from build123d import *

# Parameters (mm, degrees)
F1_DEPTH = 100
F3_DEPTH = 100.001
F5_D     = 9


with BuildPart() as f1:
    # F0 (on Top) → F1 (new body)
    with BuildSketch(Plane.XY):
        with BuildLine():
            ThreePointArc((22, 17), (20.535534, 20.535534), (17, 22))
            Line((17, 22), (-17, 22))
            ThreePointArc((-17, 22), (-20.535534, 20.535534), (-22, 17))
            Line((-22, 17), (-22, -17))
            ThreePointArc((-22, -17), (-20.535534, -20.535534), (-17, -22))
            Line((-17, -22), (17, -22))
            ThreePointArc((17, -22), (20.535534, -20.535534), (22, -17))
            Line((22, -17), (22, 17))
        make_face()
    extrude(amount=F1_DEPTH)

    # F2 (on face) → F3 (cut, through all)
    with BuildSketch(Plane.XY.offset(100)):
        with BuildLine():
            ThreePointArc((-19, -17), (-18.414214, -18.414214), (-17, -19))
            Line((-17, -19), (17, -19))
            ThreePointArc((17, -19), (18.414214, -18.414214), (19, -17))
            Line((19, -17), (19, 17))
            ThreePointArc((19, 17), (18.414214, 18.414214), (17, 19))
            Line((17, 19), (-17, 19))
            ThreePointArc((-17, 19), (-18.414214, 18.414214), (-19, 17))
            Line((-19, 17), (-19, -17))
        make_face()
    extrude(amount=-F3_DEPTH, mode=Mode.SUBTRACT)

    # F5 (through all)
    with Locations(Plane.YZ.offset(22)):
        with Locations((0, 50)):
            Hole(F5_D / 2)


solid = f1.part
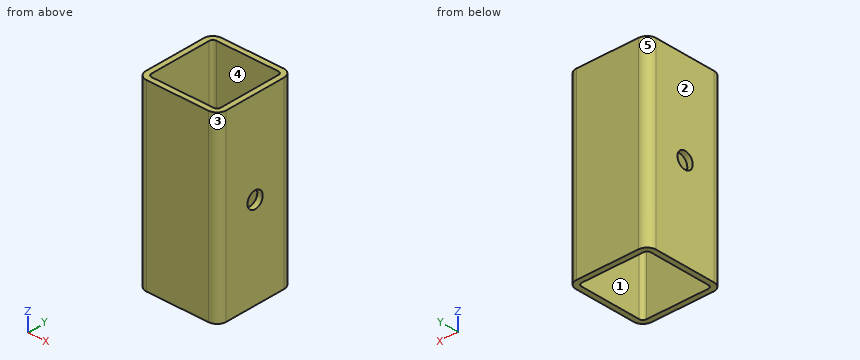
Here's how the part is built. I have some questions about the finished solid (model axes, mm). Face numbers are marked on the shaded views. A direction names the side the tool comes from. Round coordinates to 2 decimals unless told otherwise and drop trailing zeros. Write each loop counter-clockwise with the first axis right and the second up, starting at its lowest first coordinate (ties: lowest second). Pieces come first, ordered by that corner, then holes.
1. Suppose I cut it at D-D (z = 74). List the corners of the cut face in (x, y) for me.
2. For the marked faces 4 and 5, which set-ups out of +Z, -Z, +X, -X, +Y, -Y let a thin tool reach every point of the face, with its end or its side?
3. If we mould it in two halves opening along X, with no side actions, what happens to the marked faces 1, 2 and 3? For each: released by +X, released by -X, zero draft, split by the parting line, or undercut.
4. I need wall thicknesses on L1, parallel to Y at x = 15.5, z = 40; L2, parallel to Z at x = 20.6, y = 0. Which ranges of each line are inside material? Lowest first, please.
5. Suppose I cut it at B-B (y = 8.5). List the corners of the cut face in (x, z) for me.
6. Suppose I cut it at A-A (z = 50). List the corners of the cut face in (x, y) for me, and give its area (3 significant figures).
7. Will this pin go through, and if not, where does the flat tip stop? pin 1 Ø8 at (y, z) = (0, 50) entering from -X.
Answer sheet:
1. outline: (-22, -17) arc R5 ccw to (-17, -22) - (17, -22) arc R5 ccw to (22, -17) - (22, 17) arc R5 ccw to (17, 22) - (-17, 22) arc R5 ccw to (-22, 17) - close; hole (-19, -17) arc R2 ccw to (-17, -19) - (17, -19) arc R2 ccw to (19, -17) - (19, 17) arc R2 ccw to (17, 19) - (-17, 19) arc R2 ccw to (-19, 17) - close
2. face 4: +Z, -Z
2. face 5: +Z, -Z, -X, +Y
3. face 1: undercut
3. face 2: released by -X
3. face 3: released by +X
4. L1: y = -22 to -19, 19 to 22
4. L2: z = 0 to 45.5, 54.5 to 100
5. outline: (-22, 0) - (-19, 0) - (-19, 100) - (-22, 100) - close; (19, 0) - (22, 0) - (22, 100) - (19, 100) - close
6. outline: (-22, -17) arc R5 ccw to (-17, -22) - (17, -22) arc R5 ccw to (22, -17) - (22, -4.5) - (19, -4.5) - (19, -17) arc R2 cw to (17, -19) - (-17, -19) arc R2 cw to (-19, -17) - (-19, -4.5) - (-22, -4.5) - close; (-22, 4.5) - (-19, 4.5) - (-19, 17) arc R2 cw to (-17, 19) - (17, 19) arc R2 cw to (19, 17) - (19, 4.5) - (22, 4.5) - (22, 17) arc R5 ccw to (17, 22) - (-17, 22) arc R5 ccw to (-22, 17) - close
6. area: 420 mm2
7. pin 1: passes through
